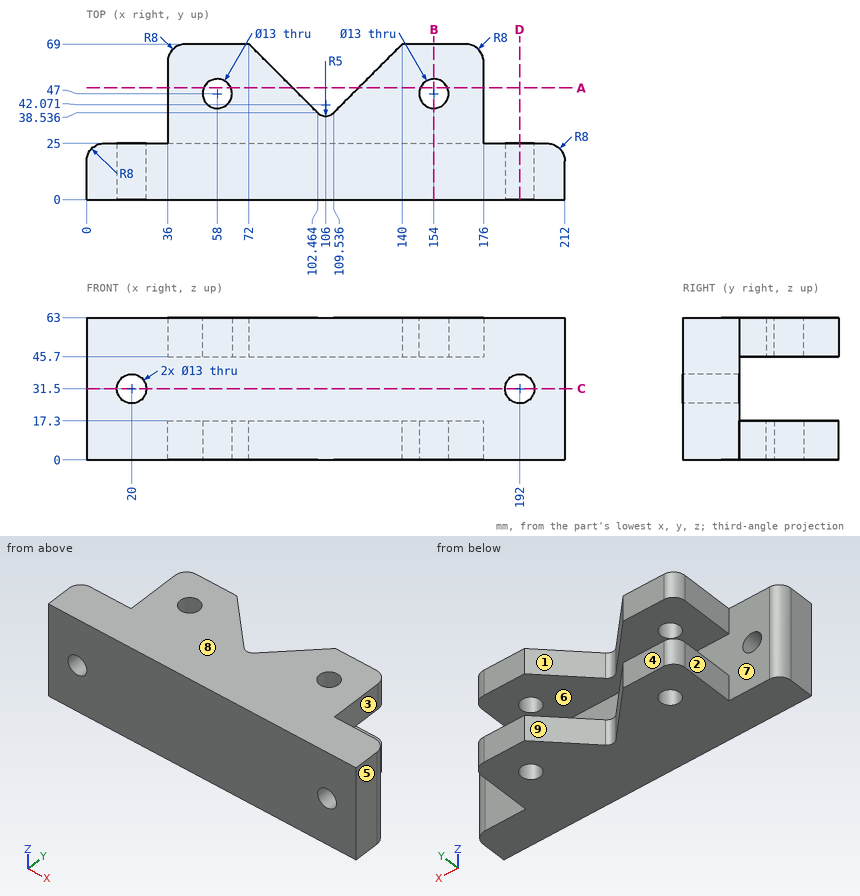
Source: three-view drawing plus pictorial views. Frame: mm from the lowest corner of the part. A direction names the side the tool comes from. Coordinates: 2 decimals unless noted, no trailing zeros. Loops run counter-clockwise (first coordinate to the right, second up) from the corner with the lowest first, then second, coordinate; pieces in that order, holes last. Notation, with made-up numbers: (2.5, 36.5) - (36.5, 36.5) arc R19 cw to (36.5, 59.5) - close; hole circle Ø9 at (84.25, 77.25). An arc over 180 degrees is marked (long way). Answer in a Markdown table with one row per item. Add a question column.
Item 1: Section query C-C on z = 31.5. Return the cut outline in (x, y).
Item 2: Section query D-D on x = 192. Return the cut outline in (y, z), then the cut area to 3 significant figures.
Item 3: Access query for the marked faces 1, 2, 3, 4 and 5. Directions: +Z, -Z, +X, -X, +Y, -Y. A direction counts if a zero-diameter tool reaches every point of the face in a straight line with its end or side. Return the directions, or none.
Item 4: Section query A-A on y = 49.5. State how many separate pieces and enclosed holes the cut face has, then the cut area to 3 significant figures.
Item 5: Contact query for flat-ended pins moving along their axis: P1, Ø14, axis at y = 46.5, z = 56.5, coming from the +X side; P2, Ø19, axis at x = 92, z = 16.5, coming from the +Y side; P3, Ø14, axis at y = 44.5, z = 52, coming from the -X side. Output: stop coordinate, or through.
Item 6: Line query: line 1 along Z through (x, y) = (144.5, 45); line 2 along Y through (x, z) = (154, 56); line 3 along X through (y, z) = (38.5, 57). Output: solid intervals per line, ascending. Write a range as [from, to].
Item 7: Mould query, pull axis Z, two halves, no side actions, for the marked faces 6, 7, 8 and 9. Classes: released by +Z, released by -Z, zero draft, split by the parting line, or undercut.
Item 8: Section query B-B on x = 154. Return the cut outline in (y, z).
Recorded:
| question | item | result |
|---|---|---|
| 1 | outline | (0, 0) - (13.5, 0) - (13.5, 25) - (8, 25) arc R8 ccw to (0, 17) - close; (26.5, 0) - (185.5, 0) - (185.5, 25) - (26.5, 25) - close; (198.5, 0) - (212, 0) - (212, 17) arc R8 ccw to (204, 25) - (198.5, 25) - close |
| 2 | outline | (0, 0) - (25, 0) - (25, 25) - (0, 25) - close; (0, 38) - (25, 38) - (25, 63) - (0, 63) - close |
| 2 | area | 1,250 mm^2 |
| 3 | face 1 | +Z, -Z, +Y |
| 3 | face 2 | +Z, -Z, -X, +Y |
| 3 | face 3 | +Z, -Z, +X, +Y |
| 3 | face 4 | +Z, -Z, +X, -X, +Y |
| 3 | face 5 | +Z, -Z, +X, +Y, -Y |
| 4 | separate pieces | 8 |
| 4 | enclosed holes | 0 |
| 4 | area | 3,010 mm^2 |
| 5 | P1 | x = 176 |
| 5 | P2 | y = 58.5 |
| 5 | P3 | x = 36 |
| 6 | line 1 | [0, 17.3], [45.7, 63] |
| 6 | line 2 | [0, 40.5], [53.5, 69] |
| 6 | line 3 | [36, 102.5], [109.5, 176] |
| 7 | face 6 | undercut |
| 7 | face 7 | undercut |
| 7 | face 8 | released by +Z |
| 7 | face 9 | zero draft |
| 8 | outline | (0, 0) - (40.5, 0) - (40.5, 17.3) - (25, 17.3) - (25, 45.7) - (40.5, 45.7) - (40.5, 63) - (0, 63) - close; (53.5, 0) - (69, 0) - (69, 17.3) - (53.5, 17.3) - close; (53.5, 45.7) - (69, 45.7) - (69, 63) - (53.5, 63) - close |
